Source: CAD feature listing. Evaluate the final solid. Frame: model axes, mm. Face numbers are marked on the shaded views. Round coordinates to 2 decimals unless told otherwise and drop trailing zeros. Write each loop counter-clockwise with the first axis right and the second up, starting at its lowest first coordinate (ties: lowest second). Pieces come first, ordered by that corner, then holes.
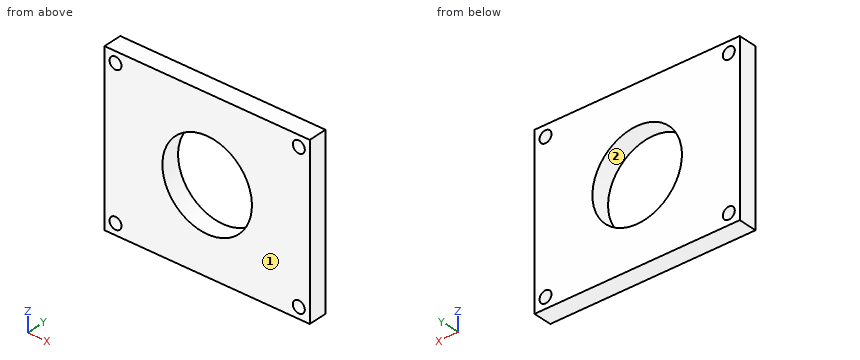
from build123d import *

# Parameters (mm, degrees)
SKETCH1_W           = 55
SKETCH1_H           = 45
BOSS_EXTRUDE1_DEPTH = 5
SKETCH2_R           = 12
CUT_EXTRUDE1_DEPTH  = 5
SKETCH3_R           = 1.6
CUT_EXTRUDE2_DEPTH  = 10


with BuildPart() as part:
    # Sketch1 → Boss-Extrude1 (new body)
    with BuildSketch(Plane(origin=(0, 0, 0), x_dir=(1, 0, 0), z_dir=(0, 1, 0))):
        with Locations((27.5, -22.5)):
            Rectangle(SKETCH1_W, SKETCH1_H)
    extrude(amount=BOSS_EXTRUDE1_DEPTH)

    # Sketch2 → Cut-Extrude1 (cut)
    with BuildSketch(Plane(origin=(0, 5, 0), x_dir=(1, 0, 0), z_dir=(0, 1, 0))):
        with Locations(Location((27.5, -22.5, 0), (0, 0, 270))):
            Circle(SKETCH2_R)
    extrude(amount=-CUT_EXTRUDE1_DEPTH, mode=Mode.SUBTRACT)

    # Sketch3 → Cut-Extrude2 (cut)
    with BuildSketch(Plane(origin=(0, 5, 0), x_dir=(1, 0, 0), z_dir=(0, 1, 0))):
        with Locations(Location((2.935211994, -2.935211994, 0), (0, 0, 270))):
            Circle(SKETCH3_R)
        with Locations(Location((52.064788006, -2.935211994, 0), (0, 0, 270))):
            Circle(SKETCH3_R)
        with Locations(Location((52.064788006, -42.064788006, 0), (0, 0, 270))):
            Circle(SKETCH3_R)
        with Locations(Location((2.935211994, -42.064788006, 0), (0, 0, 270))):
            Circle(SKETCH3_R)
    extrude(amount=-CUT_EXTRUDE2_DEPTH, mode=Mode.SUBTRACT)


solid = part.part
1) Pull-direction query (X, two-part tool) for the marked faces 1 and 2; classes: released by +X, released by -X, zero draft, split by the parting line, or undercut.
Taken from the geometry:
face 1: zero draft
face 2: undercut
2) Section query C-C on y = 4.3. Return the cut outline in (x, z).
Taken from the geometry:
outline: (0, 0) - (55, 0) - (55, 45) - (0, 45) - close; hole circle Ø3.2 at (2.94, 2.94); hole circle Ø3.2 at (2.94, 42.06); hole circle Ø24 at (27.5, 22.5); hole circle Ø3.2 at (52.06, 2.94); hole circle Ø3.2 at (52.06, 42.06)
3) Section query B-B on x = 27.5. Return the cut outline in (y, z), then the cut area to 3 significant figures.
Taken from the geometry:
outline: (0, 0) - (5, 0) - (5, 10.5) - (0, 10.5) - close; (0, 34.5) - (5, 34.5) - (5, 45) - (0, 45) - close
area: 105 mm2
4) Section query A-A on z = 22.5. Return the cut outline in (x, y), then the cut area to 3 significant figures.
Taken from the geometry:
outline: (0, 0) - (15.5, 0) - (15.5, 5) - (0, 5) - close; (39.5, 0) - (55, 0) - (55, 5) - (39.5, 5) - close
area: 155 mm2
5) Material intervals for line 1 (Z direction, x = 53, y = 1.8); line 2 (X direction, y = 2.85, z = 22.5); line 3 (X direction, y = 1.05, z = 2), sorted ascending.
Taken from the geometry:
line 1: z = 0 to 1.64, 4.23 to 40.77, 43.36 to 45
line 2: x = 0 to 15.5, 39.5 to 55
line 3: x = 0 to 1.64, 4.23 to 50.77, 53.36 to 55
